Study the drawing (mm; zero at the part's minimum x, y, z) and answer. A direction names the side the tool comes from. Round coordinates to 2 decimals unless told otherwise and drop trailing zeros. Order: outer loops, then holes, each group sorted by start corner. A loop starts at its lowest first (then second) coordinate and runs counter-clockwise, first axis right, second up. Notation, with made-up numbers: (-2.5, 32.25) - (20.5, 32.25) arc R16 cw to (20.5, 59.25) - close; hole circle Ø9 at (-5, 18). An arc over 180 degrees is marked (long way). Put each result on its own line as item: value.
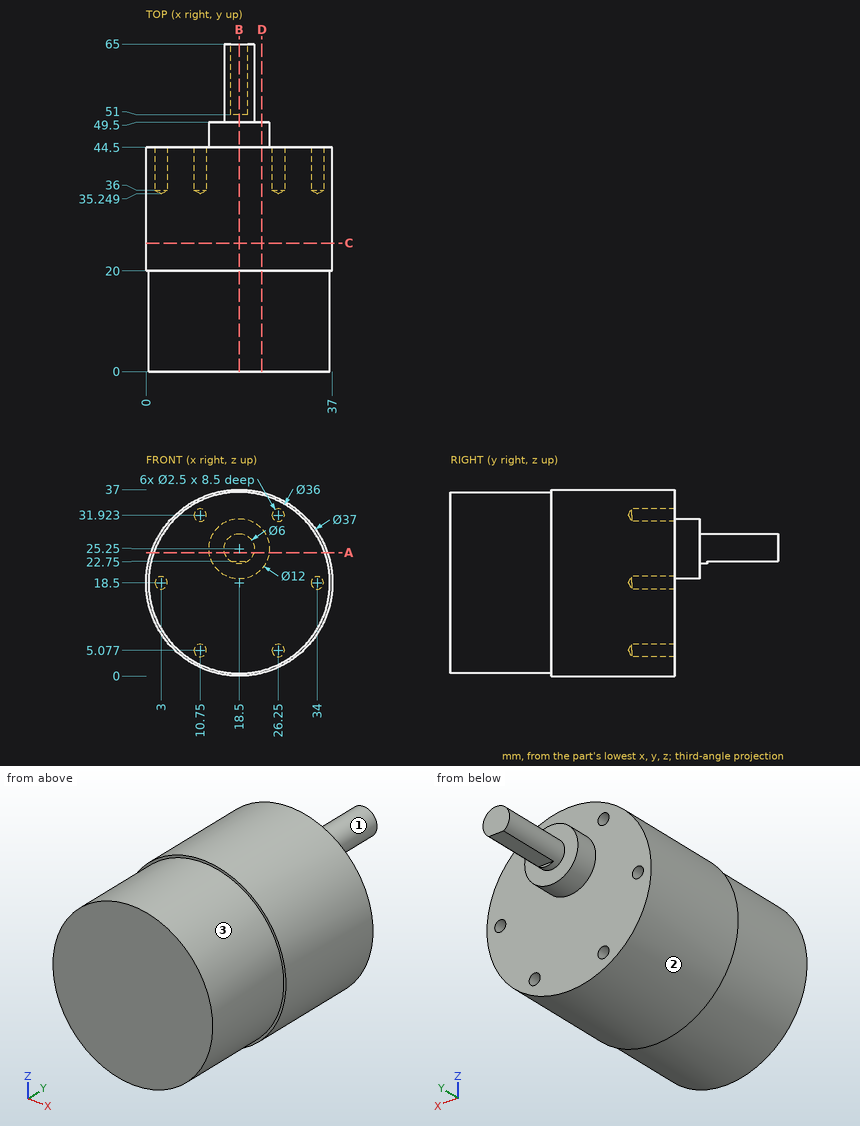
1) Straight lines are drawn through the part: L1, parallel to X at y = 41, z = 18.5; L2, parallel to X at y = 42, z = 18 (1 decimal); L3, parallel to Z at x = 26, y = 41. For each, find the intervals that lie inside material, in ascending order. Write a range as from..to.
Findings below:
L1: x = 0..1.75, 4.25..32.75, 35.25..37
L2: x = 0..1.9, 4.1..32.9, 35.1..37
L3: z = 1.59..3.85, 6.3..30.7, 33.15..35.41
2) For the marked faces 1, 2 and 3, determine the directions among +Z, -Z, +X, -X, +Y, -Y from which every point of the face is accessible in a straight line to the end or side of a thin tool.
Findings below:
face 1: +Y
face 2: +Y, -Y
face 3: -Y
3) A cutting plane is placed at A-A on z = 24.5. Write down the section's boundary in (x, y) (1 decimal).
Findings below:
outline: (1, 20) - (1.5, 20) - (1.5, 0) - (35.5, 0) - (35.5, 20) - (36, 20) - (36, 44.5) - (24.5, 44.5) - (24.5, 49.5) - (21.4, 49.5) - (21.4, 65) - (15.6, 65) - (15.6, 49.5) - (12.5, 49.5) - (12.5, 44.5) - (1, 44.5) - close
4) A cutting plane is placed at C-C on y = 25.5. Write down the section's boundary in (x, z).
Findings below:
outline: circle Ø37 at (18.5, 18.5)
5) A cutting plane is placed at D-D on x = 23. Write down the section's boundary in (y, z) (1 decimal).
Findings below:
outline: (0, 1.1) - (20, 1.1) - (20, 0.6) - (44.5, 0.6) - (44.5, 21.3) - (49.5, 21.3) - (49.5, 29.2) - (44.5, 29.2) - (44.5, 36.4) - (20, 36.4) - (20, 35.9) - (0, 35.9) - close
6) A cutting plane is placed at B-B on x = 18.5. Write down the section's boundary in (y, z), then the cut area to 3 significant figures.
Findings below:
outline: (0, 0.5) - (20, 0.5) - (20, 0) - (44.5, 0) - (44.5, 19.25) - (49.5, 19.25) - (49.5, 22.25) - (51, 22.25) - (51, 22.75) - (65, 22.75) - (65, 28.25) - (49.5, 28.25) - (49.5, 31.25) - (44.5, 31.25) - (44.5, 37) - (20, 37) - (20, 36.5) - (0, 36.5) - close
area: 1,770 mm2
7) Given pin 1 Ø1.7 at (x, y) = (18, 56) entering from -Z; pin 2 Ø3 at (x, z) = (34, 18.5) entering from +Y; pin 3 Ø12 at (y, z) = (17.5, 5) entering from -X, each flat-ended and moving along its own axis, determine where each tip first touches the part or whether it passes through.
Findings below:
pin 1: stops at z = 22.75
pin 2: stops at y = 44.5
pin 3: stops at x = 1.84
